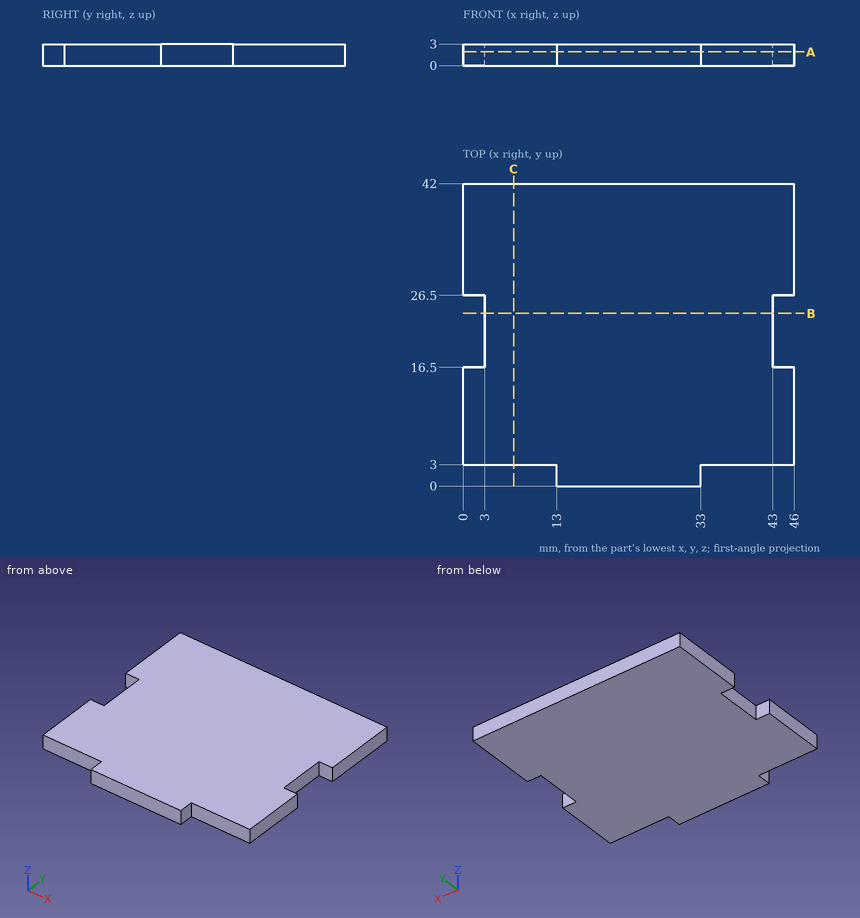
Verification items for this drawing (mm, ordinates from the low corner). Round coordinates to 2 decimals unless told otherwise and drop trailing zeros. Loops run counter-clockwise (first coordinate to the right, second up) from the corner with the lowest first, then second, coordinate; pieces in that order, holes last. Notation, with made-up numbers: (37.25, -12.75) - (60.25, -12.75) arc R6 cw to (60.25, -4.75) - close; hole circle Ø11 at (44, 8). An arc over 180 degrees is marked (long way). Answer as CSV lines item,"result". Start each with the question number.
Item 1: Section check C-C (x = 7). Record the boundary of the cut face in (y, z).
Item 2: Scan lines: line 1 (Y direction, x = 36.5, z = 0.9); line 2 (X direction, y = 19.5, z = 2.7). Record each from-to range of solid material in increasing order. Write a range as [from, to].
Item 3: Section check A-A (z = 1.9). Record the boundary of the cut face in (x, y), and give its area (3 significant figures).
Item 4: Section check B-B (y = 24). Record the boundary of the cut face in (x, z).
Item 5: Depth check by flat-ended pin: P1, Ø1.5, axis at x = 1, z = 1.5, coming from the -Y side; P2, Ø0.9, axis at y = 1, z = 1.5, coming from the +X side. Enter the tip coordinate at first touch or a pass-through.
Report:
1,outline,"(3, 0) - (42, 0) - (42, 3) - (3, 3) - close"
2,line 1,"y = [3, 42]"
2,line 2,"x = [3, 43]"
3,outline,"(0, 3) - (13, 3) - (13, 0) - (33, 0) - (33, 3) - (46, 3) - (46, 16.5) - (43, 16.5) - (43, 26.5) - (46, 26.5) - (46, 42) - (0, 42) - (0, 26.5) - (3, 26.5) - (3, 16.5) - (0, 16.5) - close"
3,area,"1,790 mm2"
4,outline,"(3, 0) - (43, 0) - (43, 3) - (3, 3) - close"
5,P1,"stops at y = 3"
5,P2,"stops at x = 33"
